Design review of the part built by this model. Coordinates are the model's own, in mm. Give positions to 0.01 mm unless a question says otherwise; leave off trailing zeros. Order: outer loops, then holes, each group sorted by start corner. A loop starts at its lowest first (then second) coordinate and runs counter-clockwise, first axis right, second up. Notation, with made-up numbers: (32, -11.75) -> (78, -11.75) arc R28 ccw to (78, 22.25) -> close; hole circle Ø2 at (60, -18.5). An arc over 180 degrees is marked (long way). One line per item, written item: value. Start each with the question number.
1) Wall thickness on line 1 along Z through (x, y) = (0.5, 218); line 2 along Z through (x, y) = (3, 129): over which ranges is each line inside the solid? List them lowest first. Write a range as from..to.
2) Consider section C-C (y = 479.5). State the section outline as (x, z) points, plus the area to 3 significant figures.
3) For pin 1 (3 mm diameter, centred on y = 505, z = -13, fed in from -X); pin 2 (8 mm diameter, centred on x = -2.5, y = 365.5, fed in from +Z); pin 3 (2 mm diameter, centred on y = 591, z = -19.5, fed in from -X); pin 4 (6 mm diameter, centred on x = 7, y = 530.5, fed in from +Z), all flat-tipped, find the tip position at first contact; note any pin that passes through.
4) Consider section B-B (z = 10.5). State the section outline as (x, y) points.
5) Consider section A-A (x = 0). State the section outline as (y, z) points, plus the area to 3 significant figures.
from build123d import *

# Parameters (mm, degrees)
SKETCH1_R           = 17.5
BOSS_EXTRUDE1_DEPTH = 600
SKETCH5_W           = 10
SKETCH5_H           = 4.03
BOSS_EXTRUDE2_DEPTH = 12


with BuildPart() as part:
    # Sketch1 → Boss-Extrude1 (new body)
    with BuildSketch(Plane(origin=(0, 0, 0), x_dir=(1, 0, 0), z_dir=(0, 1, 0))):
        Circle(SKETCH1_R)
    extrude(amount=BOSS_EXTRUDE1_DEPTH)

    # Sketch5 → Boss-Extrude2 (add)
    with BuildSketch(Plane(origin=(0, 600, 0), x_dir=(1, 0, 0), z_dir=(0, 1, 0))):
        with Locations((0, 18.78551)):
            Rectangle(SKETCH5_W, SKETCH5_H)
    extrude(amount=-BOSS_EXTRUDE2_DEPTH)


solid = part.part
Checked values:
1. line 1: z = -17.49..17.49
1. line 2: z = -17.24..17.24
2. outline: circle Ø35 at (0, 0)
2. area: 962 mm^2
3. pin 1: stops at x = -13.19
3. pin 2: stops at z = 17.5
3. pin 3: stops at x = -5
3. pin 4: stops at z = 17.04
4. outline: (-14, 0) -> (14, 0) -> (14, 600) -> (-14, 600) -> close
5. outline: (0, -17.5) -> (588, -17.5) -> (588, -20.8) -> (600, -20.8) -> (600, 17.5) -> (0, 17.5) -> close
5. area: 21,000 mm^2
